Read the model definition and answer for the solid it produces. Units are mm, in the model's axes. Face numbers are marked on the shaded views. Coordinates: 2 decimals unless noted, no trailing zeros. Order: outer loops, then holes, each group sorted by start corner. A loop starts at its lowest first (then second) coordinate and runs counter-clockwise, first axis right, second up. Notation, with made-up numbers: M 14,68 L 18,68 A10 cw 18,85 Z; hole C -5,-10 d4. An arc over 180 degrees is marked long. Use a Markdown table: item, result. Add a question column.
1) Each of these flat-tipped pins is pushed along its axis until it touches: pin 1 Ø1 at (y, z) = (77, 8) entering from -X; pin 2 Ø1.2 at (x, z) = (150.5, 1) entering from +Y; pin 3 Ø3 at (x, y) = (118.5, 47) entering from +Z. Where does it stop, or does it pass through?
2) The mould has two halves that part along Z. Classify the marked faces 1 and 2: released by +Z, released by -Z, zero draft, split by the parting line, or undercut.
3) Find the intervals of material crossed by probe 1 along Y at (x, z) = (246.38, 0.3); probe 2 along Y at (x, z) = (264.16, 1.2); probe 3 along Z at (x, y) = (187.5, 26), in increasing order. Write a range as [from, to].
4) Find section C-C on z = 12.25. Write down the section's boundary in (x, y).
5) Find section A-A on x = 79. Write down the section's boundary in (y, z).
6) Find section B-B on y = 79. Write down the section's boundary in (x, z).
7) Find section D-D on x = 310.5. Write down the section's boundary in (y, z).
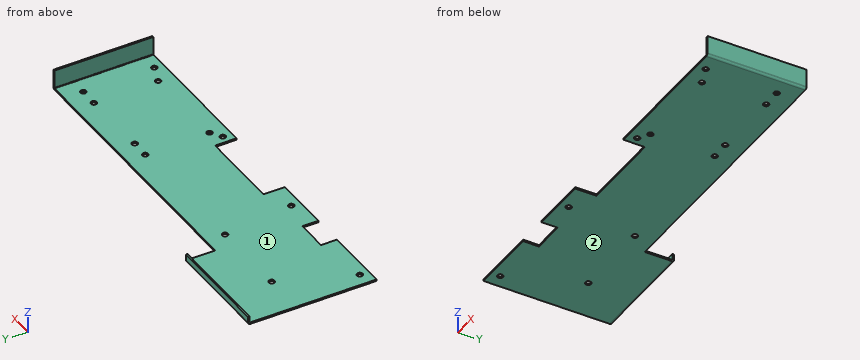
from build123d import *

# Parameters (mm, degrees)
BASE_FLANGE1_DEPTH    = 1.524
MITER_START           = -3.608291964
MITER_FLANGE1_DEPTH   = 93.967487941
MITER_FLANGE1_2_DEPTH = 93.967487941
MITER_FLANGE2_DEPTH   = 101.6
MITER_FLANGE2_2_DEPTH = 101.6
SKETCH6_R             = 2.7051
PCB_MOUNT_HOLES_DEPTH = 2.54
SKETCH7_W             = 78.994
SKETCH7_H             = 20.32
SKETCH7_W_2           = 30.48
SKETCH7_H_2           = 15.24
CUT_EXTRUDE2_DEPTH    = 2.54
SKETCH8_R             = 2.7051
CUT_EXTRUDE3_DEPTH    = 2.54
LPATTERN1_COUNT       = 2
LPATTERN1_PITCH       = 83.82
LPATTERN1_COUNT_DIR2  = 2
LPATTERN1_PITCH_DIR2  = 60.96


# Read off the part's stored shape, not the designer's step: Miter Flange1, Miter Flange2
# Sheet-metal steps are written as plain solids
with BuildPart() as part:
    # Sketch1 → Base-Flange1 (new body)
    with BuildSketch(Plane.XY):
        Polygon((0, 0), (0, -3.608291964), (365.76, -3.608291964), (365.76, 90.359195977), (254, 90.359195977), (254, 90.371708036), (101.6, 90.371708036), (101.6, 118.311708036), (0, 118.311708036), align=None)
    extrude(amount=BASE_FLANGE1_DEPTH)

    # Miter Flange1 outline → Miter Flange1 (cut)
    with BuildSketch(Plane(origin=(0, 0, 0), x_dir=(1, 0, 0), z_dir=(0, 1, 0)).offset(MITER_START)):
        with BuildLine():
            ThreePointArc((363.4994, 0), (364.811869886, -0.420019885), (365.636625492, -1.524))
            Line((365.636625492, -1.524), (365.76, -1.524))
            Line((365.76, -1.524), (365.76, 0))
            Line((365.76, 0), (363.4994, 0))
        make_face()
    extrude(amount=MITER_FLANGE1_DEPTH, mode=Mode.SUBTRACT)

    # Miter Flange1 2 outline → Miter Flange1 2 (add)
    with BuildSketch(Plane(origin=(0, 0, 0), x_dir=(1, 0, 0), z_dir=(0, 1, 0)).offset(MITER_START)):
        with BuildLine():
            Line((364.236, -19.304), (365.76, -19.304))
            Line((365.76, -19.304), (365.76, -2.2606))
            ThreePointArc((365.76, -2.2606), (365.728943037, -1.887169675), (365.636625492, -1.524))
            Line((365.636625492, -1.524), (363.4994, -1.524))
            ThreePointArc((363.4994, -1.524), (364.020254855, -1.739745145), (364.236, -2.2606))
            Line((364.236, -2.2606), (364.236, -19.304))
        make_face()
    extrude(amount=MITER_FLANGE1_2_DEPTH)

    # Miter Flange2 outline → Miter Flange2 (cut)
    with BuildSketch(Plane.YZ):
        with BuildLine():
            Line((118.311708036, 1.524), (118.188333528, 1.524))
            ThreePointArc((118.188333528, 1.524), (117.363577922, 0.420019885), (116.051108036, 0))
            Line((116.051108036, 0), (118.311708036, 0))
            Line((118.311708036, 0), (118.311708036, 1.524))
        make_face()
    extrude(amount=MITER_FLANGE2_DEPTH, mode=Mode.SUBTRACT)

    # Miter Flange2 2 outline → Miter Flange2 2 (add)
    with BuildSketch(Plane.YZ):
        with BuildLine():
            Line((118.311708036, 7.62), (116.787708036, 7.62))
            Line((116.787708036, 7.62), (116.787708036, 2.2606))
            ThreePointArc((116.787708036, 2.2606), (116.571962891, 1.739745145), (116.051108036, 1.524))
            Line((116.051108036, 1.524), (118.188333528, 1.524))
            ThreePointArc((118.188333528, 1.524), (118.280651073, 1.887169675), (118.311708036, 2.2606))
            Line((118.311708036, 2.2606), (118.311708036, 7.62))
        make_face()
    extrude(amount=MITER_FLANGE2_2_DEPTH)

    # Sketch6 → PCB mount holes (cut)
    with BuildSketch(Plane.XY.offset(1.524)):
        with Locations((347.98, 4.926108036)):
            Circle(SKETCH6_R)
        with Locations((347.98, 72.236108036)):
            Circle(SKETCH6_R)
        with Locations((264.16, 72.236108036)):
            Circle(SKETCH6_R)
        with Locations((236.22, 4.926108036)):
            Circle(SKETCH6_R)
        with Locations((12.7, 4.926108036)):
            Circle(SKETCH6_R)
        with Locations((40.64, 72.236108036)):
            Circle(SKETCH6_R)
        with Locations((116.84, 72.236108036)):
            Circle(SKETCH6_R)
        with Locations((124.46, 4.926108036)):
            Circle(SKETCH6_R)
    extrude(amount=-PCB_MOUNT_HOLES_DEPTH, mode=Mode.SUBTRACT)

    # Sketch7 → Cut-Extrude2 (cut)
    with BuildSketch(Plane.XY.offset(1.524)):
        with Locations((189.103, 6.551708036)):
            Rectangle(SKETCH7_W, SKETCH7_H)
        with Locations((79.756, 4.011708036)):
            Rectangle(SKETCH7_W_2, SKETCH7_H_2)
    extrude(amount=-CUT_EXTRUDE2_DEPTH, mode=Mode.SUBTRACT)

    # Sketch8 → Cut-Extrude3 (cut)
    with BuildSketch(Plane.XY.offset(1.524)):
        with Locations((330.2, 11.631708036)):
            Circle(SKETCH8_R)
    cut_extrude3 = extrude(amount=-CUT_EXTRUDE3_DEPTH, mode=Mode.SUBTRACT)

    # LPattern1: Cut-Extrude3 2 × 2
    with Locations(*[(-i * LPATTERN1_PITCH, j * LPATTERN1_PITCH_DIR2, 0) for i in range(LPATTERN1_COUNT) for j in range(LPATTERN1_COUNT_DIR2) if (i, j) != (0, 0)]):
        add(cut_extrude3, mode=Mode.SUBTRACT)


solid = part.part
Check result:
| question | item | result |
|---|---|---|
| 1 | pin 1 | stops at x = 364.24 |
| 1 | pin 2 | stops at y = 90.37 |
| 1 | pin 3 | stops at z = 1.52 |
| 2 | face 1 | released by +Z |
| 2 | face 2 | released by -Z |
| 3 | probe 1 | y = [-3.61, 8.93], [14.34, 69.89], [75.3, 90.37] |
| 3 | probe 2 | y = [-3.61, 69.53], [74.94, 90.36] |
| 3 | probe 3 | z = [0, 1.52] |
| 4 | outline | M 364.24,-3.61 L 365.76,-3.61 L 365.76,90.36 L 364.24,90.36 Z |
| 5 | outline | M 11.63,0 L 116.05,0 A2.26 ccw 118.31,2.26 L 118.31,7.62 L 116.79,7.62 L 116.79,2.26 A0.74 cw 116.05,1.52 L 11.63,1.52 Z |
| 6 | outline | M 0,0 L 363.5,0 A2.26 ccw 365.76,2.26 L 365.76,19.3 L 364.24,19.3 L 364.24,2.26 A0.74 cw 363.5,1.52 L 0,1.52 Z |
| 7 | outline | M -3.61,0 L 90.36,0 L 90.36,1.52 L -3.61,1.52 Z |
